Source: CAD feature listing. Evaluate the final solid. Frame: model axes, mm. A direction names the side the tool comes from. Round coordinates to 2 decimals unless told otherwise and drop trailing zeros. Write each loop counter-clockwise with the first axis right and the second up, starting at its lowest first coordinate (ties: lowest second). Pieces come first, ordered by that corner, then holes. Notation, with made-up numbers: M 55,16.5 L 93,16.5 A21 ccw 93,40.5 Z; hole C 50.25,-15.5 d2. An arc over 180 degrees is marked long. Use a Markdown table: item, result.
```python
from build123d import *

# Parameters (mm, degrees)
F2_DEPTH = 76.2
F3_DEPTH = 41.275


with BuildPart() as f2:
    # F1 (on Right) → F2 (new body)
    with BuildSketch(Plane.YZ):
        Polygon((-38.0939699973, 0.2813866025), (-3.175, -319.0764911919), (0, -325.4264911919), (3.175, -319.0764911919), (38.0939699973, 0.2813866025), align=None)
        with BuildLine():
            ThreePointArc((38.0939699973, 0.2813866025), (0, 17.4735088081), (-38.0939699973, 0.2813866025))
            Line((-38.0939699973, 0.2813866025), (38.0939699973, 0.2813866025))
        make_face()
    extrude(amount=F2_DEPTH)

    # F0 (on Front) → F3 (join, symmetric)
    with BuildSketch(Plane.XZ):
        with BuildLine():
            Line((59.4184325825, -215.8783343432), (59.4184325825, 1.3118497446))
            ThreePointArc((59.4184325825, 1.3118497446), (30.8434325825, 16.1563866025), (2.2684325825, 1.3118497446))
            Line((2.2684325825, 1.3118497446), (2.2684325825, -215.8783343432))
            Line((2.2684325825, -215.8783343432), (20.5285961914, -326.7436133975))
            Line((20.5285961914, -326.7436133975), (41.1582689735, -326.7436133975))
            Line((41.1582689735, -326.7436133975), (59.4184325825, -215.8783343432))
        make_face()
        with BuildLine():
            ThreePointArc((5.4434325825, 0.2813866025), (30.8434325825, 12.9813866025), (56.2434325825, 0.2813866025))
            Line((56.2434325825, 0.2813866025), (56.2434325825, -215.6186133975))
            Line((56.2434325825, -215.6186133975), (38.4634325825, -323.5686133975))
            Line((38.4634325825, -323.5686133975), (23.2234325825, -323.5686133975))
            Line((23.2234325825, -323.5686133975), (5.4434325825, -215.6186133975))
            Line((5.4434325825, -215.6186133975), (5.4434325825, 0.2813866025))
        make_face(mode=Mode.SUBTRACT)
    extrude(amount=F3_DEPTH, both=True)


solid = f2.part
```
Q1. Section A-A on y = -27. Return loops of the section in (x, z) (3 decimals), plus the area to 3 significant figures.
Results are:
| item | result |
|---|---|
| outline | M 0,-101.181 L 2.268,-101.181 L 2.268,-215.878 L 20.529,-326.744 L 41.158,-326.744 L 59.418,-215.878 L 59.418,-101.181 L 76.2,-101.181 L 76.2,9.704 L 51.069,9.704 A34.925 ccw 10.618,9.704 L 0,9.704 Z; hole M 5.443,-215.619 L 23.223,-323.569 L 38.463,-323.569 L 56.243,-215.619 L 56.243,-101.181 L 5.443,-101.181 Z; hole M 16.795,9.704 L 44.892,9.704 A31.75 ccw Z |
| area | 10,100 mm^2 |
Q2. First-contact query: pin 1 Ø6 at (x, z) = (9.5, -291.5) entering from +Y; pin 2 Ø4.5 at (x, y) = (34.5, 14) entering from +Z; pin 3 Ø10 at (x, y) = (37.5, -9.5) entering from +Z. Flat tips, straight axial feed; report the tip coordinate or a pass-through.
Results are:
| item | result |
|---|---|
| pin 1 | y = 6.52 |
| pin 2 | z = 16.13 |
| pin 3 | z = 17.27 |
Q3. Reachability of faces 4 (the flat face through (56.243, -31, -130)), 5 (the flat face through (59.418, 31, -133)), 6 (the flat face through (5.443, 31, -133)), 7 (the flat face through (10.01, -1.61, -322.21)) from +Z, -Z, +X, -X, +Y, -Y: full face, straight path, thin tool, end or side. Return the list, or none.
Results are:
| item | result |
|---|---|
| face 4 | -Y |
| face 5 | -Z, +X, +Y |
| face 6 | +Y |
| face 7 | -Z, -X, -Y |
Q4. Section B-B on x = 46. Return loops of the section in (y, z) (1 decimal), plus the area to 3 significant figures.
Results are:
| item | result |
|---|---|
| outline | M -41.3,-297.3 L -5.6,-297.3 L -3.2,-319.1 L 0,-325.4 L 3.2,-319.1 L 5.6,-297.3 L 41.3,-297.3 L 41.3,-277.8 L 7.7,-277.8 L 38.1,0.3 A50.8 ccw 27.9,9.1 L 41.3,9.1 L 41.3,12.7 L 21.5,12.7 A50.8 ccw -21.5,12.7 L -41.3,12.7 L -41.3,9.1 L -27.9,9.1 A50.8 ccw -38.1,0.3 L -7.7,-277.8 L -41.3,-277.8 Z |
| area | 15,600 mm^2 |
Q5. Section D-D on y = 33.5. Return loops of the section in (x, z) (3 decimals).
Results are:
| item | result |
|---|---|
| outline | M 0,-41.734 L 2.268,-41.734 L 2.268,-215.878 L 20.529,-326.744 L 41.158,-326.744 L 59.418,-215.878 L 59.418,-41.734 L 76.2,-41.734 L 76.2,4.862 L 56.56,4.862 A34.925 ccw 5.127,4.862 L 0,4.862 Z; hole M 5.443,-215.619 L 23.223,-323.569 L 38.463,-323.569 L 56.243,-215.619 L 56.243,-41.734 L 5.443,-41.734 Z; hole M 9.639,4.862 L 52.048,4.862 A31.75 ccw Z |
Q6. Line query: L1, parallel to X at y = 22.5, z = -182.5; L2, parallel to X at y = -32, z = -248.5; L3, parallel to Y at x = 61.5, z = 0. Output: solid intervals per line, ascending.
Results are:
| item | result |
|---|---|
| L1 | 2.27 to 5.44, 56.24 to 59.42 |
| L2 | 7.64 to 10.86, 50.83 to 54.05 |
| L3 | -38.06 to 38.06 |
Q7. Mould query, pull axis Z, two halves, no side actions, for faces 1 (the flat face through (31, -1, -326.744)), 2 (the flat face through (14.46, 25.3, -270.35)), 3 (the cylindrical face through (31.312, -29.888, 16.153)). Classes: +Z half, -Z half, draft (parallel to the pull), parting line (faces both ways), or undercut.
Results are:
| item | result |
|---|---|
| face 1 | -Z half |
| face 2 | undercut |
| face 3 | +Z half |
Q8. Section C-C on z = -11.5. Return loops of the section in (x, y) (3 decimals).
Results are:
| item | result |
|---|---|
| outline | M 0,-36.806 L 2.268,-36.806 L 2.268,-41.275 L 5.443,-41.275 L 5.443,-36.806 L 56.243,-36.806 L 56.243,-41.275 L 59.418,-41.275 L 59.418,-36.806 L 76.2,-36.806 L 76.2,36.806 L 59.418,36.806 L 59.418,41.275 L 56.243,41.275 L 56.243,36.806 L 5.443,36.806 L 5.443,41.275 L 2.268,41.275 L 2.268,36.806 L 0,36.806 Z |
